Check sheet for the drawn part. Datum: minimum x, y, z corner. Units: mm. A direction names the side the tool comes from. Coordinates: 2 decimals unless noted, no trailing zeros. Write each loop counter-clockwise with the first axis right and the second up, starting at its lowest first coordinate (ties: lowest second). Pieces come first, ordered by that corner, then holes. Notation, with made-up numbers: M 63.5,14.5 L 105.5,14.5 A17 cw 105.5,23.5 Z; hole C 37.5,80.5 d1. An arc over 180 degrees is marked long. Answer in a Markdown table with one row per item.
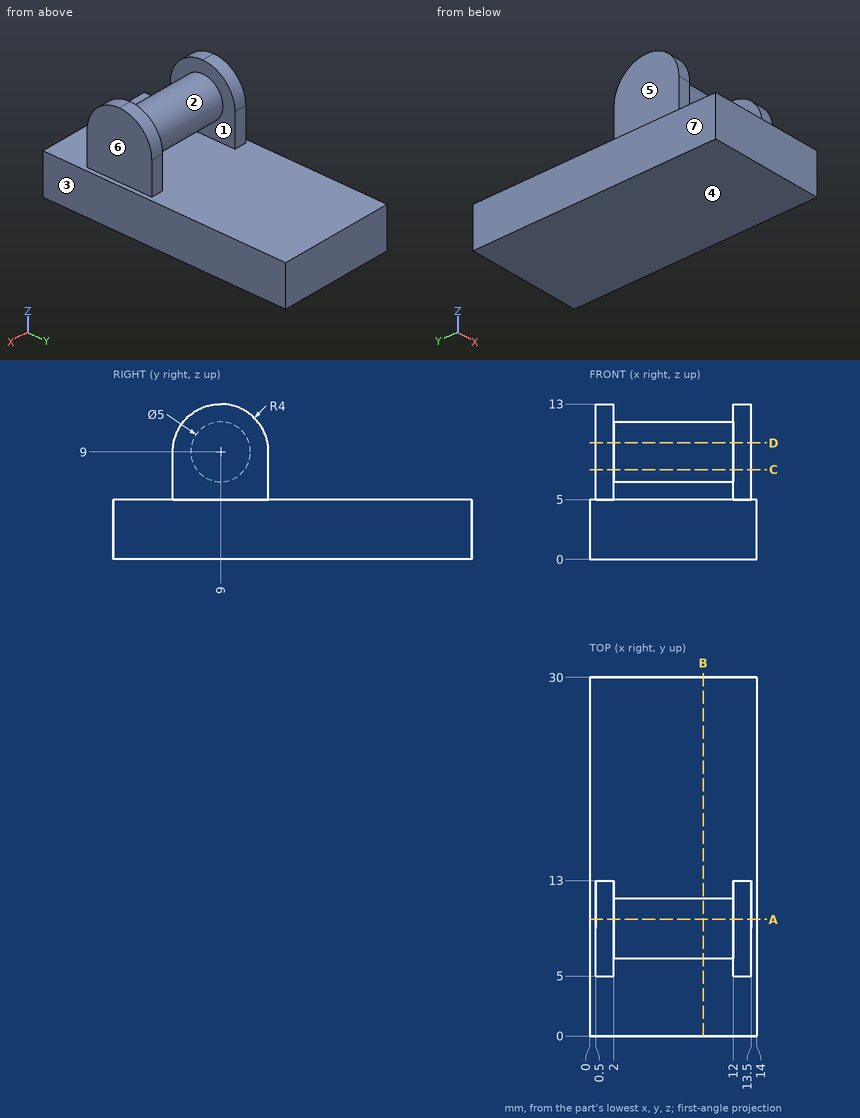
1) Thickness scan on L1, parallel to X at y = 12.75, z = 10; L2, parallel to Y at x = 12.25, z = 6; L3, parallel to Z at x = 1.25, y = 19. Record the ranges inside material, lowest first. Write a range as [from, to].
Response values:
| item | result |
|---|---|
| L1 | x = [0.5, 2], [12, 13.5] |
| L2 | y = [5, 13] |
| L3 | z = [0, 5] |
2) Tool access check on the marked faces 5, 6 and 7. Record the directions out of +Z, -Z, +X, -X, +Y, -Y that give a thin tool (end or side, any length) a straight path to the whole face; none if there is none.
Response values:
| item | result |
|---|---|
| face 5 | +Z, -X, +Y, -Y |
| face 6 | +Z, +X, +Y, -Y |
| face 7 | +Z, -Z, -X, +Y, -Y |
3) Sectioned sample at C-C (z = 7.5). Record the cut outline in (x, y).
Response values:
| item | result |
|---|---|
| outline | M 0.5,5 L 2,5 L 2,7 L 12,7 L 12,5 L 13.5,5 L 13.5,13 L 12,13 L 12,11 L 2,11 L 2,13 L 0.5,13 Z |
4) Sectioned sample at D-D (z = 9.75). Record the cut outline in (x, y), then the cut area to 3 significant figures.
Response values:
| item | result |
|---|---|
| outline | M 0.5,5.07 L 2,5.07 L 2,6.62 L 12,6.62 L 12,5.07 L 13.5,5.07 L 13.5,12.93 L 12,12.93 L 12,11.38 L 2,11.38 L 2,12.93 L 0.5,12.93 Z |
| area | 71.3 mm² |
5) Depth check by flat-ended pin: pin 1 (1.2 mm diameter, centred on x = 12.5, z = 8, fed in from -Y); pin 2 (1.2 mm diameter, centred on x = 1, z = 7.5, fed in from +Y); pin 3 (6.5 mm diameter, centred on y = 7.5, z = 10.5, fed in from +X); pin 4 (1 mm diameter, centred on x = 4, y = 9.5, fed in from -Z). Enter the tip coordinate at first touch or a pass-through.
Response values:
| item | result |
|---|---|
| pin 1 | stops at y = 5 |
| pin 2 | stops at y = 13 |
| pin 3 | stops at x = 13.5 |
| pin 4 | stops at z = 0 |
6) Release check for a two-part mould opening along Z. For the marked faces 1, 2, 3 and 4 record: +Z half, -Z half, draft (parallel to the pull), parting line (faces both ways), or undercut.
Response values:
| item | result |
|---|---|
| face 1 | undercut |
| face 2 | undercut |
| face 3 | draft |
| face 4 | -Z half |
7) Sectioned sample at B-B (x = 9.5). Record the cut outline in (y, z), then the cut area to 3 significant figures.
Response values:
| item | result |
|---|---|
| outline | M 0,0 L 30,0 L 30,5 L 0,5 Z; C 9,9 d5 |
| area | 170 mm² |
8) Sectioned sample at A-A (y = 9.75). Record the cut outline in (x, z), then the cut area to 3 significant figures.
Response values:
| item | result |
|---|---|
| outline | M 0,0 L 14,0 L 14,5 L 13.5,5 L 13.5,12.93 L 12,12.93 L 12,11.38 L 2,11.38 L 2,12.93 L 0.5,12.93 L 0.5,5 L 0,5 Z; hole M 2,5 L 12,5 L 12,6.62 L 2,6.62 Z |
| area | 141 mm² |
